Work out the finished part from the listing and answer in its coordinate system (mm). A direction names the side the tool comes from. Round coordinates to 2 decimals unless told otherwise and drop trailing zeros. Loops run counter-clockwise (first coordinate to the right, second up) from the corner with the lowest first, then second, coordinate; pieces in that order, holes last. Notation, with made-up numbers: (24.25, 27) -> (82.25, 27) arc R12 ccw to (82.25, 47) -> close; hole circle Ø2 at (-23.5, 26). An arc over 180 degrees is marked (long way). Use CSV: the item, a comma, the result in double quotes. Start each with the question number.
from build123d import *

# Parameters (mm, degrees)
BOSS_EXTRU_2_DEPTH      = 18
ENL_V_MAT_EXTRU_1_DEPTH = 19
CONG_1_R                = 7


with BuildPart() as part:
    # Esquisse2 → Boss.-Extru.2 (new body)
    with BuildSketch(Plane.XY):
        with BuildLine():
            Line((0, 0), (100, 0))
            Line((100, 0), (100, 46.012238509))
            ThreePointArc((100, 46.012238509), (99.874827529, 46.793387794), (99.511844635, 47.496314371))
            ThreePointArc((99.511844635, 47.496314371), (100, 54), (106.503685629, 54.488155365))
            ThreePointArc((106.503685629, 54.488155365), (107.206612206, 54.125172471), (107.987761491, 54))
            Line((107.987761491, 54), (157.994949366, 54))
            Line((157.994949366, 54), (157.994949366, 360))
            Line((157.994949366, 360), (-30, 360))
            Line((-30, 360), (-30, 54))
            Line((-30, 54), (-7.987761491, 54))
            ThreePointArc((-7.987761491, 54), (-7.206612206, 54.125172471), (-6.503685629, 54.488155365))
            ThreePointArc((-6.503685629, 54.488155365), (0, 54), (0.488155365, 47.496314371))
            ThreePointArc((0.488155365, 47.496314371), (0.125172471, 46.793387794), (0, 46.012238509))
            Line((0, 46.012238509), (0, 0))
        make_face()
    extrude(amount=BOSS_EXTRU_2_DEPTH)

    # Esquisse1 → Enlèv. mat.-Extru.1 (cut, through all)
    with BuildSketch(Plane.XY):
        with BuildLine():
            Line((59.5, 28.248771852), (59.5, 25.751228148))
            ThreePointArc((59.5, 25.751228148), (59.599672829, 25.160561143), (59.88765279, 24.635309084))
            ThreePointArc((59.88765279, 24.635309084), (59.5, 18), (52.864690916, 17.61234721))
            ThreePointArc((52.864690916, 17.61234721), (52.339438857, 17.900327171), (51.748771852, 18))
            Line((51.748771852, 18), (48.251228148, 18))
            ThreePointArc((48.251228148, 18), (47.660561143, 17.900327171), (47.135309084, 17.61234721))
            ThreePointArc((47.135309084, 17.61234721), (40.5, 18), (40.11234721, 24.635309084))
            ThreePointArc((40.11234721, 24.635309084), (40.400327171, 25.160561143), (40.5, 25.751228148))
            Line((40.5, 25.751228148), (40.5, 28.248771852))
            ThreePointArc((40.5, 28.248771852), (40.400327171, 28.839438857), (40.11234721, 29.364690916))
            ThreePointArc((40.11234721, 29.364690916), (40.5, 36), (47.135309084, 36.38765279))
            ThreePointArc((47.135309084, 36.38765279), (47.660561143, 36.099672829), (48.251228148, 36))
            Line((48.251228148, 36), (51.748771852, 36))
            ThreePointArc((51.748771852, 36), (52.339438857, 36.099672829), (52.864690916, 36.38765279))
            ThreePointArc((52.864690916, 36.38765279), (59.5, 36), (59.88765279, 29.364690916))
            ThreePointArc((59.88765279, 29.364690916), (59.599672829, 28.839438857), (59.5, 28.248771852))
        make_face()
    extrude(amount=ENL_V_MAT_EXTRU_1_DEPTH, mode=Mode.SUBTRACT)

    # Congé1
    cong_1_edges = [part.edges().sort_by_distance(p)[0] for p in [
        (-30, 54, 9),
        (157.994949366, 54, 9),
        (100, 0, 9),
        (0, 0, 9),
    ]]
    fillet(cong_1_edges, radius=CONG_1_R)

    # Symétrie1: part across plane


with BuildPart() as part_1:
    add(part.part)
    add(part.part.mirror(Plane(origin=(157.994949366, 360, 18), x_dir=(0, 0, 1), z_dir=(0, -1, 0))))


solid = part_1.part
Q1. Straight lines are drawn through the part: line 1 (Y direction, x = -0.5, z = 15); line 2 (Y direction, x = 119.5, z = 7.5); line 3 (X direction, y = 686, z = 2.75). For each, find the intervals that lie inside material, in ascending order. Write a range as from..to.
Q2. Which of the six approach directions +Z, -Z, +X, -X, +Y, -Y give full straight-line access (tool end or side, diameter ignored) to faces 1 (the flat face through (100, 694, 9)), 2 (the flat face through (100, 26, 9)), 3 (the flat face through (0, 693, 9))?
Q3. Each of these flat-tipped pins is pushed along its axis until it touches: pin 1 (9 mm diameter, centred on x = 125.5, z = 10.5, fed in from +Y); pin 2 (2.5 mm diameter, centred on y = 693, z = 11, fed in from -X); pin 3 (2 mm diameter, centred on y = 693.5, z = 9.5, fed in from +X). Where does it stop, or does it pass through?
Q4. Section A-A, the plane z = 3 is taken. Give the number of separate pieces and of enclosed holes in the cut face, and give its area (3 significant figures).
Q5. Section B-B, the plane x = 136 is taken. Write down the section's boundary in (y, z).
Report:
1,line 1,"y = 54.44..665.56"
1,line 2,"y = 54..666"
1,line 3,"x = 0..39.28, 60.72..100"
2,face 1,"+Z, -Z, +X, +Y"
2,face 2,"+Z, -Z, +X, -Y"
2,face 3,"+Z, -Z, -X, +Y"
3,pin 1,"stops at y = 666"
3,pin 2,"stops at x = 0"
3,pin 3,"stops at x = 100"
4,separate pieces,"1"
4,enclosed holes,"2"
4,area,"125,000 mm²"
5,outline,"(54, 0) -> (666, 0) -> (666, 18) -> (54, 18) -> close"
